```python
from build123d import *

# Parameters (mm, degrees)
F1_DEPTH = 70
F4_DEPTH = 75.001


with BuildPart() as f1:
    # F0 (on Front) → F1 (new body)
    with BuildSketch(Plane.XZ):
        Polygon((0, 75), (0, 0), (125, 0), (125, 75), (95, 75), (95, 55), (25, 55), (25, 75), align=None)
    extrude(amount=F1_DEPTH)

    # F3 (on offset) → F4 (cut, through all)
    with BuildSketch(Plane.XY.offset(75)):
        Polygon((50, -55), (0, -55), (0, -70), (105, -70), (105, -42.5), (80, -42.5), (80, -40), (50, -40), align=None)
    extrude(amount=-F4_DEPTH, mode=Mode.SUBTRACT)


solid = f1.part
```
Input: part model. Units: mm. Frame: model coordinates. A direction names the side the tool comes from. Give positions to 0.01 mm unless a question says otherwise; leave off trailing zeros. Order: outer loops, then holes, each group sorted by start corner. A loop starts at its lowest first (then second) coordinate and runs counter-clockwise, first axis right, second up. Notation, with made-up numbers: (35.5, -14) - (47.5, -14) arc R25 ccw to (47.5, 14) - close; hole circle Ø1 at (-8.75, 29). An arc over 180 degrees is marked (long way). Put each result on its own line as item: value.
Item 1: Section query C-C, the plane z = 50.5. Return loops of the section in (x, y), then the cut area to 3 significant figures.
Found:
outline: (0, -55) - (50, -55) - (50, -40) - (80, -40) - (80, -42.5) - (105, -42.5) - (105, -70) - (125, -70) - (125, 0) - (0, 0) - close
area: 6,410 mm^2
Item 2: Section query B-B, the plane y = -49. Return loops of the section in (x, z).
Found:
outline: (0, 0) - (50, 0) - (50, 55) - (25, 55) - (25, 75) - (0, 75) - close; (105, 0) - (125, 0) - (125, 75) - (105, 75) - close
Item 3: Draft query along X for faces 1 (the flat face through (0, -27, 38)), 2 (the flat face through (110, -35, 75)), 3 (the flat face through (105, -56, 38)). Return one class per face: +X half, -X half, draft (parallel to the pull), parting line (faces both ways), or undercut.
Found:
face 1: -X half
face 2: draft
face 3: undercut
Item 4: Ray query, L1, parallel to X at y = -22.5, z = 55.5; L2, parallel to X at y = -41.5, z = 24; L3, parallel to Y at x = 5, z = 46.5. Return the intervals inside material, ascending. Write a range as from..to.
Found:
L1: x = 0..25, 95..125
L2: x = 0..50, 80..125
L3: y = -55..0
Item 5: Section query D-D, the plane y = -24.5. Return loops of the section in (x, z).
Found:
outline: (0, 0) - (125, 0) - (125, 75) - (95, 75) - (95, 55) - (25, 55) - (25, 75) - (0, 75) - close
Item 6: Access query for faces 4 (the flat face through (60, -21, 55)), 5 (the flat face through (25, -55, 38)), 6 (the flat face through (93, -42.5, 38)). Directions: +Z, -Z, +X, -X, +Y, -Y. A direction counts if a zero-diameter tool reaches every point of the face in a straight line with its end or side. Return the directions, or none.
Found:
face 4: +Z, +Y, -Y
face 5: +Z, -Z, -X, -Y
face 6: +Z, -Z, -Y
Item 7: Section query A-A, the plane z = 67. Return loops of the section in (x, y).
Found:
outline: (0, -55) - (25, -55) - (25, 0) - (0, 0) - close; (95, -42.5) - (105, -42.5) - (105, -70) - (125, -70) - (125, 0) - (95, 0) - close
Item 8: Contact query for flat-ended pins moving along their axis: pin 1 (7.5 mm diameter, centred on x = 88, z = 26, fed in from -Y); pin 2 (12 mm diameter, centred on x = 39, y = -23, fed in from +Z); pin 3 (1.5 mm diameter, centred on y = -57, z = 22, fed in from -X). Output: stop coordinate, or through.
Found:
pin 1: stops at y = -42.5
pin 2: stops at z = 55
pin 3: stops at x = 105
